For this review, take the finished solid that the model builds, in its own axes (mm). A direction names the side the tool comes from. Give positions to 0.01 mm unless a question says otherwise; leave off trailing zeros. Order: outer loops, then holes, each group sorted by start corner. A loop starts at its lowest first (then second) coordinate and runs counter-clockwise, first axis right, second up.
Item 1: The part is to be moulded in two halves that separate along Z. For faces 1 (the flat face through (3, -38, -20)), 2 (the cylindrical face through (1.521, -57.513, -12.305)), 3 (the flat face through (1, -56, 0)), say which applies: released by +Z, released by -Z, zero draft, split by the parting line, or undercut.
Item 2: Consider section D-D (z = -56). Give the boundary of the cut face in (x, y).
Item 3: Consider section B-B (z = -12.5). Give the boundary of the cut face in (x, y), plus the area to 3 significant figures.
Item 4: Consider section C-C (x = 1.2). Give the boundary of the cut face in (y, z).
Item 5: For probe 1 along Y at (x, z) = (1.75, -12.5); probe 2 along Y at (x, z) = (1.5, -60.5); probe 3 along Z at (x, y) = (1.75, -11.5), list the stretches that pass through material, from the lowest coordinate up.
Item 6: Machinability: for faces 4 (the flat face through (2, -65, -25)), 5 (the cylindrical face through (1.521, -81.513, -12.305)), which of the approach directions +Z, -Z, +X, -X, +Y, -Y give a long, thin tool a straight path to every point of the face, cutting with its end or side? Answer none if there is none.
Item 7: Consider section A-A (y = -83). Give the boundary of the cut face in (x, z).
Item 8: For P1, Ø1.5, axis at x = 1.5, y = -65.5, coming from the -Z side; P2, Ø1.8, axis at y = -11, z = -60.5, coming from the +X side; P3, Ø1, axis at x = 2, y = -25.5, coming from the -Z side, all flat-tipped, find the tip position at first contact; note any pin that passes through.
```python
from build123d import *

# Parameters (mm, degrees)
CROQUIS1_W              = 75
CROQUIS1_H              = 100
SALIENTE_EXTRUIR1_DEPTH = 3
CROQUIS2_W              = 50
CROQUIS2_H              = 80
CORTAR_EXTRUIR1_DEPTH   = 3
REDONDEO1_R             = 10
REDONDEO3_R             = 5
CROQUIS3_R              = 1.5
CORTAR_EXTRUIR2_DEPTH   = 3


with BuildPart() as part:
    # Croquis1 → Saliente-Extruir1 (new body)
    with BuildSketch(Plane(origin=(0, 0, 0), x_dir=(0, 0, -1), z_dir=(1, 0, 0))):
        with Locations((37.5, -50)):
            Rectangle(CROQUIS1_W, CROQUIS1_H)
    extrude(amount=SALIENTE_EXTRUIR1_DEPTH)

    # Croquis2 → Cortar-Extruir1 (cut)
    with BuildSketch(Plane(origin=(3, 0, 0), x_dir=(0, 0, -1), z_dir=(1, 0, 0))):
        with Locations((50, -60)):
            Rectangle(CROQUIS2_W, CROQUIS2_H)
    extrude(amount=-CORTAR_EXTRUIR1_DEPTH, mode=Mode.SUBTRACT)

    # Redondeo1
    redondeo1_edges = [part.edges().sort_by_distance(p)[0] for p in [
        (1.5, -20, -25),
        (1.5, 0, 0),
    ]]
    fillet(redondeo1_edges, radius=REDONDEO1_R)

    # Redondeo3
    redondeo3_edges = [part.edges().sort_by_distance(p)[0] for p in [
        (1.5, -20, -75),
        (1.5, 0, -75),
    ]]
    fillet(redondeo3_edges, radius=REDONDEO3_R)

    # Croquis3 → Cortar-Extruir2 (cut)
    with BuildSketch(Plane(origin=(3, 0, 0), x_dir=(0, 0, -1), z_dir=(1, 0, 0))):
        with Locations((12.5, -11)):
            Circle(CROQUIS3_R)
        with Locations((12.5, -59)):
            Circle(CROQUIS3_R)
        with Locations((12.5, -83)):
            Circle(CROQUIS3_R)
        with Locations((12.5, -35)):
            Circle(CROQUIS3_R)
        with Locations((36.5, -11)):
            Circle(CROQUIS3_R)
        with Locations((60.5, -11)):
            Circle(CROQUIS3_R)
    extrude(amount=-CORTAR_EXTRUIR2_DEPTH, mode=Mode.SUBTRACT)


solid = part.part
```
Resolved:
1. face 1: zero draft
1. face 2: undercut
1. face 3: released by +Z
2. outline: (0, -20) - (3, -20) - (3, 0) - (0, 0) - close
3. outline: (0, -100) - (3, -100) - (3, -84.5) - (0, -84.5) - close; (0, -81.5) - (3, -81.5) - (3, -60.5) - (0, -60.5) - close; (0, -57.5) - (3, -57.5) - (3, -36.5) - (0, -36.5) - close; (0, -33.5) - (3, -33.5) - (3, -12.5) - (0, -12.5) - close; (0, -9.5) - (3, -9.5) - (3, 0) - (0, 0) - close
3. area: 264 mm2
4. outline: (-100, -25) - (-30, -25) arc R10 cw to (-20, -35) - (-20, -70) arc R5 ccw to (-15, -75) - (-5, -75) arc R5 ccw to (0, -70) - (0, -10) arc R10 ccw to (-10, 0) - (-100, 0) - close; hole circle Ø3 at (-83, -12.5); hole circle Ø3 at (-59, -12.5); hole circle Ø3 at (-35, -12.5); hole circle Ø3 at (-11, -60.5); hole circle Ø3 at (-11, -36.5); hole circle Ø3 at (-11, -12.5)
5. probe 1: y = -100 to -84.5, -81.5 to -60.5, -57.5 to -36.5, -33.5 to -12.5, -9.5 to 0
5. probe 2: y = -20 to -12.5, -9.5 to 0
5. probe 3: z = -75 to -61.91, -59.09 to -37.91, -35.09 to -13.91, -11.09 to 0
6. face 4: -Z, +X, -X, -Y
6. face 5: +X, -X
7. outline: (0, -25) - (3, -25) - (3, -14) - (0, -14) - close; (0, -11) - (3, -11) - (3, 0) - (0, 0) - close
8. P1: stops at z = -25
8. P2: passes through
8. P3: stops at z = -26.34
